from build123d import *

# Parameters (mm, degrees)
SKETCH1_W           = 25.4
SKETCH1_H           = 50.8
SKETCH1_W_2         = 22.225
SKETCH1_H_2         = 47.625
BOSS_EXTRUDE1_DEPTH = 127


with BuildPart() as part:
    # Sketch1 → Boss-Extrude1 (new, symmetric)
    with BuildSketch(Plane(origin=(0, 0, 0), x_dir=(0, 0, -1), z_dir=(1, 0, 0))):
        with Locations((1.923003206, 0)):
            Rectangle(SKETCH1_W, SKETCH1_H)
        with Locations((1.923003206, 0)):
            Rectangle(SKETCH1_W_2, SKETCH1_H_2, mode=Mode.SUBTRACT)
    extrude(amount=BOSS_EXTRUDE1_DEPTH, both=True)


solid = part.part
CAD build for the part. Positions are in the model's coordinates, mm. A direction names the side the tool comes from. Coordinates: 2 decimals unless noted, no trailing zeros. Write each loop counter-clockwise with the first axis right and the second up, starting at its lowest first coordinate (ties: lowest second). Pieces come first, ordered by that corner, then holes. Notation, with made-up numbers: (52, -31) - (106, -31) arc R9 ccw to (106, -19) - close; hole circle Ø3 at (48.25, 1.5). An arc over 180 degrees is marked (long way). Use a Markdown table: item, result. Add a question column.
Item 1: Flat gauge pin, fed straight in: pin 1 (6 mm diameter, centred on y = 18.5, z = -4.5, fed in from -X). Where does the tip first touch, or does it go through?
Item 2: Band-saw the part on C-C, the plane z = 6. Give the cut face in (x, y), and give its area (3 significant figures).
Item 3: Band-saw the part on A-A, the plane x = -109. Give the cut face in (y, z).
Item 4: 3-axis set-ups, long thin cutter, end or side, ignore diameter. For faces 4 (the face through (2, -23.812, -2)), 5 (the face through (-127, 2, 9.4)): which of +Z, -Z, +X, -X, +Y, -Y reach the whole face in a straight line?
Item 5: Drill centre lines: L1, parallel to Y at x = 89, z = -11.25; L2, parallel to Z at x = 7, y = 10. Where is each one in solid material? Low to high. Write a range as from..to.
Item 6: Band-saw the part on B-B, the plane y = 6.5. Give the cut face in (x, z), and give its area (3 significant figures).
Item 7: Mould opens along Y. For faces 1 (the face through (2, -25.4, -2)), 2 (the face through (2, 23.812, -2)), 3 (the face through (127, 2, 9.4)) say: pulls with the +Y half, pulls with the -Y half, needs draft (parallel to the pull), parting line crosses it, or undercut.
Numbers:
| question | item | result |
|---|---|---|
| 1 | pin 1 | through |
| 2 | outline | (-127, -25.4) - (127, -25.4) - (127, -23.81) - (-127, -23.81) - close; (-127, 23.81) - (127, 23.81) - (127, 25.4) - (-127, 25.4) - close |
| 2 | area | 806 mm2 |
| 3 | outline | (-25.4, -14.62) - (25.4, -14.62) - (25.4, 10.78) - (-25.4, 10.78) - close; hole (-23.81, -13.04) - (23.81, -13.04) - (23.81, 9.19) - (-23.81, 9.19) - close |
| 4 | face 4 | +X, -X |
| 4 | face 5 | +Z, -Z, -X, +Y, -Y |
| 5 | L1 | -25.4..-23.81, 23.81..25.4 |
| 5 | L2 | -14.62..-13.04, 9.19..10.78 |
| 6 | outline | (-127, -14.62) - (127, -14.62) - (127, -13.04) - (-127, -13.04) - close; (-127, 9.19) - (127, 9.19) - (127, 10.78) - (-127, 10.78) - close |
| 6 | area | 806 mm2 |
| 7 | face 1 | pulls with the -Y half |
| 7 | face 2 | undercut |
| 7 | face 3 | needs draft |
